from build123d import *

# Parameters (mm, degrees)
SKETCH1_R             = 2.75
BOSS_EXTRUDE1_DEPTH   = 8
CROQUIS1_R            = 4
CORTAR_EXTRUIR1_DEPTH = 27.874709301
CROQUIS2_W            = 0.5
CROQUIS2_H            = 20
CORTAR_EXTRUIR2_DEPTH = 27.874709301
SKETCH3_R             = 2
CUT_EXTRUDE1_DEPTH    = 33.74522866


with BuildPart() as part:
    # Sketch1 → Boss-Extrude1 (new body)
    with BuildSketch(Plane(origin=(0, 0, 0), x_dir=(1, 0, 0), z_dir=(0, 1, 0))):
        with BuildLine():
            Line((0, 14), (0, -10))
            ThreePointArc((0, -10), (-1.812396329, -9.834389638), (-3.564762336, -9.343043909))
            Line((-3.564762336, -9.343043909), (-21.5, -2.5))
            Line((-21.5, -2.5), (-21.5, 2.5))
            Line((-21.5, 2.5), (-7, 8.032356947))
            Line((-7, 8.032356947), (-7, 14))
            Line((-7, 14), (0, 14))
        make_face()
        with Locations(Location((-15, 0, 0), (0, 0, 270))):
            Circle(SKETCH1_R, mode=Mode.SUBTRACT)
    boss_extrude1 = extrude(amount=BOSS_EXTRUDE1_DEPTH)

    # Simetría1: Boss-Extrude1 across plane
    add(boss_extrude1.mirror(Plane(origin=(0, 8, -14), x_dir=(0, 0, 1), z_dir=(-1, 0, 0))))

    # Croquis1 → Cortar-Extruir1 (cut, through all)
    with BuildSketch(Plane(origin=(0, 0, 0), x_dir=(1, 0, 0), z_dir=(0, 1, 0))):
        with Locations(Location((0, 0, 0), (0, 0, 270))):
            Circle(CROQUIS1_R)
    extrude(amount=CORTAR_EXTRUIR1_DEPTH, mode=Mode.SUBTRACT)

    # Croquis2 → Cortar-Extruir2 (cut, through all)
    with BuildSketch(Plane(origin=(0, 0, 0), x_dir=(1, 0, 0), z_dir=(0, 1, 0))):
        with Locations((0, 10)):
            Rectangle(CROQUIS2_W, CROQUIS2_H)
    extrude(amount=CORTAR_EXTRUIR2_DEPTH, mode=Mode.SUBTRACT)

    # Sketch3 → Cut-Extrude1 (cut, through all)
    with BuildSketch(Plane(origin=(7, 0, 0), x_dir=(0, 0, -1), z_dir=(1, 0, 0))):
        with Locations((11, 4)):
            Circle(SKETCH3_R)
    extrude(amount=-CUT_EXTRUDE1_DEPTH, mode=Mode.SUBTRACT)


solid = part.part
Part model, mm, in its own coordinate system. A direction names the side the tool comes from. Coordinates: 2 decimals unless noted, no trailing zeros. Order: outer loops, then holes, each group sorted by start corner. A loop starts at its lowest first (then second) coordinate and runs counter-clockwise, first axis right, second up. Notation, with made-up numbers: M 56.5,89 L 90.5,89 A20 ccw 90.5,109 Z; hole C 46.5,13 d2. An arc over 180 degrees is marked long. Use a Markdown table: item, result.
(1) Tool access for faces 5 (the flat face through (7, 5, -9)), 6 (the flat face through (-7, 5, -9)), 7 (the flat face through (4, 4, -14)), 8 (the flat face through (-0.25, 4, -8)): list every direction of +Z, -Z, +X, -X, +Y, -Y with a clear straight run to the whole face (end or side of a thin tool).
A:
| item | result |
|---|---|
| face 5 | -Z, +X, +Y, -Y |
| face 6 | -Z, -X, +Y, -Y |
| face 7 | -Z, +X, -X, +Y, -Y |
| face 8 | -Z, +Y, -Y |
(2) Cut at A-A on y = 4. Write the cut outline in (x, z).
A:
| item | result |
|---|---|
| outline | M -21.5,-2.5 L -7,-8.03 L -7,-9 L -0.25,-9 L -0.25,-3.99 A4 cw long 0.25,-3.99 L 0.25,-9 L 7,-9 L 7,-8.03 L 21.5,-2.5 L 21.5,2.5 L 3.56,9.34 A10 ccw -3.56,9.34 L -21.5,2.5 Z; M -7,-14 L -0.25,-14 L -0.25,-13 L -7,-13 Z; M 0.25,-14 L 7,-14 L 7,-13 L 0.25,-13 Z; hole C -15,0 d5.5; hole C 15,0 d5.5 |
(3) Cut at D-D on x = 13. Write the cut outline in (y, z), then the cut area to 3 significant figures.
A:
| item | result |
|---|---|
| outline | M 0,-5.74 L 8,-5.74 L 8,-1.89 L 0,-1.89 Z; M 0,1.89 L 8,1.89 L 8,5.74 L 0,5.74 Z |
| area | 61.7 mm^2 |
(4) Flat gauge pins, fed straight in: pin 1 (2.5 mm diameter, centred on y = 4, z = -11, fed in from +X); pin 2 (3 mm diameter, centred on y = 3.5, z = -12, fed in from +X); pin 3 (2 mm diameter, centred on x = 9, y = 6.5, fed in from -Z). Where does each tip first touch, or does it go through?
A:
| item | result |
|---|---|
| pin 1 | passes through |
| pin 2 | stops at x = 7 |
| pin 3 | stops at z = -7.65 |
(5) Cut at B-B on z = 0. Write the cut outline in (x, y), then the cut area to 3 significant figures.
A:
| item | result |
|---|---|
| outline | M -21.5,0 L -17.75,0 L -17.75,8 L -21.5,8 Z; M -12.25,0 L -4,0 L -4,8 L -12.25,8 Z; M 4,0 L 12.25,0 L 12.25,8 L 4,8 Z; M 17.75,0 L 21.5,0 L 21.5,8 L 17.75,8 Z |
| area | 192 mm^2 |
(6) Pull direction X, two halves, no side cores. Call faces 1 (the flat face through (0.25, 4, -8)), 2 (the cylindrical face through (-12.273, 3.944, -0.358)), 3 (the flat face through (-5, 0, -2)), 4 (the flat face through (21.5, 4, 0)): released by +X, released by -X, zero draft, split by the parting line, or undercut.
A:
| item | result |
|---|---|
| face 1 | undercut |
| face 2 | undercut |
| face 3 | zero draft |
| face 4 | released by +X |
(7) Probe L1, parallel to X at y = 3.75, z = 0; L2, parallel to X at y = 1.5, z = -1; L3, parallel to Z at x = -3, y = 2.5. List the from-to ranges inside material, lowest first.
A:
| item | result |
|---|---|
| L1 | x = -21.5 to -17.75, -12.25 to -4, 4 to 12.25, 17.75 to 21.5 |
| L2 | x = -21.5 to -17.56, -12.44 to -3.87, 3.87 to 12.44, 17.56 to 21.5 |
| L3 | z = -14 to -12.32, -9.68 to -2.65, 2.65 to 9.54 |
(8) Cut at C-C on x = 3. Write the cut outline in (y, z), then the cut area to 3 significant figures.
A:
| item | result |
|---|---|
| outline | M 0,-14 L 8,-14 L 8,-2.65 L 0,-2.65 Z; M 0,2.65 L 8,2.65 L 8,9.54 L 0,9.54 Z; hole C 4,-11 d4 |
| area | 133 mm^2 |
